```python
from build123d import *

# Parameters (mm, degrees)
BOSS_EXTRUDE1_DEPTH = 50.8
FILLET1_R           = 10
SHELL1_T            = -5.08
SKETCH3_R           = 31.75
CUT_EXTRUDE2_DEPTH  = 125.434078933


with BuildPart() as part:
    # Sketch2 → Boss-Extrude1 (new body)
    with BuildSketch(Plane.XY):
        with BuildLine():
            Line((-50.8, 0), (-50.8, -101.6))
            Line((-50.8, -101.6), (50.8, -101.6))
            Line((50.8, -101.6), (50.8, 0))
            ThreePointArc((50.8, 0), (0, 50.8), (-50.8, 0))
        make_face()
    extrude(amount=BOSS_EXTRUDE1_DEPTH)

    # Fillet1
    fillet1_edges = [part.edges().sort_by_distance(p)[0] for p in [
        (50.8, -50.8, 50.8),
        (0, 50.8, 50.8),
        (-50.8, -50.8, 50.8),
    ]]
    fillet(fillet1_edges, radius=FILLET1_R)

    # Shell1
    shell1_openings = [part.faces().sort_by_distance(p)[0] for p in [
        (0, -30.396611795, 0),
    ]]
    offset(amount=SHELL1_T, openings=shell1_openings, kind=Kind.INTERSECTION)

    # Sketch3 → Cut-Extrude2 (cut, through all)
    with BuildSketch(Plane.XY.offset(50.8)):
        Circle(SKETCH3_R)
    extrude(amount=-CUT_EXTRUDE2_DEPTH, mode=Mode.SUBTRACT)


solid = part.part
```
Design review of the part built by this model. Coordinates are the model's own, in mm. A direction names the side the tool comes from. Round coordinates to 2 decimals unless told otherwise and drop trailing zeros. Order: outer loops, then holes, each group sorted by start corner. A loop starts at its lowest first (then second) coordinate and runs counter-clockwise, first axis right, second up. Notation, with made-up numbers: M 59.25,-26.75 L 64.25,-26.75 A17 ccw 64.25,-2.75 Z; hole C 41,58.5 d3. An arc over 180 degrees is marked long. Put each result on its own line as item: value.
Q1. To check wall thickness, follow line 1 (X direction, y = -32, z = 10); line 2 (Z direction, x = -35.5, y = 13); line 3 (Y direction, x = 0, z = 46.8). State the ranges of each line that lie inside material, in increasing order.
Reported:
line 1: -50.8 to -45.72, 45.72 to 50.8
line 2: 45.72 to 50.8
line 3: -101.6 to -31.75, 31.75 to 48.8
Q2. Draft analysis for pull direction Y (two halves, no side actions). For faces 1 (the face through (-49, -31, 0)), 2 (the face through (-1, -96.52, 23)), 3 (the face through (1.117, 50.788, 20.114)), state which applies: released by +Y, released by -Y, zero draft, split by the parting line, or undercut.
Reported:
face 1: zero draft
face 2: undercut
face 3: released by +Y
Q3. Machinability: for faces 4 (the face through (-44.32, -48.94, 44.24)), 5 (the face through (-1, -101.6, 25)), which of the approach directions +Z, -Z, +X, -X, +Y, -Y give a long, thin tool a straight path to every point of the face, cutting with its end or side? Answer none if there is none.
Reported:
face 4: -Z
face 5: +Z, -Z, +X, -X, -Y
Q4. Insertion check: pin 1 Ø12 at (x, z) = (-7.5, 30) entering from +Y; pin 2 Ø8 at (x, y) = (10.5, 27) entering from -Z; pin 3 Ø4 at (x, z) = (-40.5, 38.5) entering from +Y. Each pin has a flat end and moves straight along its axis. Give the tip position at first contact, or say it passes through.
Reported:
pin 1: y = 50.78
pin 2: z = 45.72
pin 3: y = 33.14
Q5. Consider section B-B (z = 8.5). State the section outline as (x, y) points.
Reported:
outline: M -50.8,-101.6 L 50.8,-101.6 L 50.8,0 A50.8 ccw -50.8,0 Z; hole M -45.72,-96.52 L 45.72,-96.52 L 45.72,0 A45.72 ccw -45.72,0 Z
Q6. Consider section C-C (y = -39). State the section outline as (x, z) points, and give its area (3 significant figures).
Reported:
outline: M -50.8,0 L -45.72,0 L -45.72,40.8 A4.92 cw -40.8,45.72 L 40.8,45.72 A4.92 cw 45.72,40.8 L 45.72,0 L 50.8,0 L 50.8,40.8 A10 ccw 40.8,50.8 L -40.8,50.8 A10 ccw -50.8,40.8 Z
area: 948 mm²
Q7. Consider section A-A (x = 0). State the section outline as (y, z) points.
Reported:
outline: M -101.6,0 L -96.52,0 L -96.52,45.72 L -31.75,45.72 L -31.75,50.8 L -101.6,50.8 Z; M 31.75,45.72 L 40.8,45.72 A4.92 cw 45.72,40.8 L 45.72,0 L 50.8,0 L 50.8,40.8 A10 ccw 40.8,50.8 L 31.75,50.8 Z
